from build123d import *

# Parameters (mm, degrees)
F0_W     = 19.05
F0_H     = 34.29
F1_DEPTH = 6.35
F2_W     = 19.05
F2_H     = 6.35
F3_DEPTH = 25.4
F4_R     = 0.5
F5_DEPTH = 6.35


with BuildPart() as f1:
    # F0 (on Front) → F1 (new body)
    with BuildSketch(Plane.XZ):
        with Locations((0, 8.08)):
            Rectangle(F0_W, F0_H)
        with BuildLine():
            ThreePointArc((-3.5, -5), (-6, 0), (-3.5, 5))
            Line((-3.5, 5), (3.5, 5))
            ThreePointArc((3.5, 5), (6, 0), (3.5, -5))
            Line((3.5, -5), (-3.5, -5))
        make_face(mode=Mode.SUBTRACT)
    extrude(amount=F1_DEPTH)

    # F2 (on face) → F3 (join)
    with BuildSketch(Plane.XZ.offset(6.35)):
        with Locations((0, 22.05)):
            Rectangle(F2_W, F2_H)
    extrude(amount=F3_DEPTH)

    # F4 (on face) → F5 (cut, through all)
    with BuildSketch(Plane.XY.offset(25.225)):
        with Locations((-8.0899, -21.30044)):
            Circle(F4_R)
        with Locations((0, -29.39034)):
            Circle(F4_R)
        with Locations((8.0899, -21.30044)):
            Circle(F4_R)
        with Locations((0, -13.21054)):
            Circle(F4_R)
    extrude(amount=-F5_DEPTH, mode=Mode.SUBTRACT)


solid = f1.part
Design review of the part built by this model. Coordinates are the model's own, in mm. A direction names the side the tool comes from. Coordinates: 2 decimals unless noted, no trailing zeros. Write each loop counter-clockwise with the first axis right and the second up, starting at its lowest first coordinate (ties: lowest second). Pieces come first, ordered by that corner, then holes. Notation, with made-up numbers: (80.5, 6) - (102.5, 6) arc R23 cw to (102.5, 22) - close; hole circle Ø2 at (62, 66). An arc over 180 degrees is marked (long way). Use one line per item in the form item = value.
Q1. Consider section C-C (y = -25.5). Write out the cut boundary in (x, z) (3 decimals).
Taken from the geometry:
outline = (-9.525, 18.875) - (9.525, 18.875) - (9.525, 25.225) - (-9.525, 25.225) - close
Q2. Consider section B-B (x = -2.5). Write out the cut boundary in (y, z) (3 decimals), plus the area to 3 significant figures.
Taken from the geometry:
outline = (-31.75, 18.875) - (-6.35, 18.875) - (-6.35, 5) - (0, 5) - (0, 25.225) - (-31.75, 25.225) - close; (-6.35, -9.065) - (0, -9.065) - (0, -5) - (-6.35, -5) - close
area = 316 mm^2
Q3. Insertion check: pin 1 Ø2 at (x, z) = (-5, 4.5) entering from -Y; pin 2 Ø5.5 at (x, y) = (-2, -18) entering from -Z (3 decimals); pin 3 Ø8 at (x, z) = (2.5, -4.5) entering from +Y. Each pin has a flat end and moves straight along its axis. Give the tip position at first contact, or say it passes through.
Taken from the geometry:
pin_1 = -6.35
pin_2 = 18.875
pin_3 = 0
Q4. For probe 1 along Y at (x, z) = (0, 23.25); probe 2 along Z at (x, y) = (-5.5, -19) (3 decimals); probe 3 along Y at (x, z) = (7.25, -1), list the stretches that pass through material, from the lowest coordinate up.
Taken from the geometry:
probe_1 = -31.75 to -29.89, -28.89 to -13.71, -12.71 to 0
probe_2 = 18.875 to 25.225
probe_3 = -6.35 to 0
Q5. Consider section A-A (x = 0). Write out the cut boundary in (y, z) (3 decimals), plus the area to 3 significant figures.
Taken from the geometry:
outline = (-31.75, 18.875) - (-29.89, 18.875) - (-29.89, 25.225) - (-31.75, 25.225) - close; (-28.89, 18.875) - (-13.711, 18.875) - (-13.711, 25.225) - (-28.89, 25.225) - close; (-12.711, 18.875) - (-6.35, 18.875) - (-6.35, 5) - (0, 5) - (0, 25.225) - (-12.711, 25.225) - close; (-6.35, -9.065) - (0, -9.065) - (0, -5) - (-6.35, -5) - close
area = 303 mm^2
Q6. The part is to be moulded in two halves that separate along Y. For faces 1 (the cylindrical face through (6, -3, 0)), 2 (the cylindrical face through (8.025, -20.805, 22.094)), 3 (the cylindrical face through (-0.11, -29.88, 22.09)), 4 (the flat face through (0, -31.75, 22)), say which applies: +Y half, -Y half, draft (parallel to the pull), parting line (faces both ways), or undercut.
Taken from the geometry:
face_1 = draft
face_2 = undercut
face_3 = undercut
face_4 = -Y half
Q7. Consider section D-D (z = 17). Write out the cut boundary in (x, y) (3 decimals), plus the area to 3 significant figures.
Taken from the geometry:
outline = (-9.525, -6.35) - (9.525, -6.35) - (9.525, 0) - (-9.525, 0) - close
area = 121 mm^2
Q8. Machinability: for faces 5 (the cylindrical face through (-6, -3, 0)), 6 (the flat face through (0, 0, 8)), 7 (the flat face through (0, -19, 18.875)), which of the approach directions +Z, -Z, +X, -X, +Y, -Y give a long, thin tool a straight path to every point of the face, cutting with its end or side? Answer none if there is none.
Taken from the geometry:
face_5 = +Y, -Y
face_6 = +Z, -Z, +X, -X, +Y
face_7 = -Z, +X, -X, -Y
